Source: CAD feature listing. Evaluate the final solid. Frame: model axes, mm. Face numbers are marked on the shaded views. Round coordinates to 2 decimals unless told otherwise and drop trailing zeros. Loops run counter-clockwise (first coordinate to the right, second up) from the corner with the lowest first, then second, coordinate; pieces in that order, holes last.
(1) Section A-A, the plane y = 0. Return the cut outline in (x, z), plus the area to 4 significant figures.
(2) Mould query, pull axis X, two halves, no side actions, for the marked faces 1, 2, 3 and 4. Classes: pulls with the +X half, pulls with the -X half, needs draft (parallel to the pull), parting line crosses it, or undercut.
(3) Material intervals for probe 1 along Y at (x, z) = (0, -3); probe 2 along Z at (x, y) = (-27, -42); probe 3 along X at (y, z) = (25, -0.5), sorted ascending.
```python
from build123d import *

# Parameters (mm, degrees)
F1_DEPTH = 30
F2_R     = 75
F2_R_2   = 65
F3_DEPTH = 5


with BuildPart() as f1:
    # F0 (on Top) → F1 (new body)
    with BuildSketch(Plane.XY):
        with BuildLine():
            ThreePointArc((98.5, 75.5), (91.763456, 91.763456), (75.5, 98.5))
            Line((75.5, 98.5), (-75.5, 98.5))
            ThreePointArc((-75.5, 98.5), (-91.763456, 91.763456), (-98.5, 75.5))
            Line((-98.5, 75.5), (-98.5, -75.5))
            ThreePointArc((-98.5, -75.5), (-91.763456, -91.763456), (-75.5, -98.5))
            Line((-75.5, -98.5), (75.5, -98.5))
            ThreePointArc((75.5, -98.5), (91.763456, -91.763456), (98.5, -75.5))
            Line((98.5, -75.5), (98.5, 75.5))
        make_face()
    extrude(amount=F1_DEPTH)

    # F2 (on face) → F3 (join)
    with BuildSketch(Plane.XY):
        with BuildLine():
            Line((98.5, -75.5), (98.5, 75.5))
            ThreePointArc((98.5, 75.5), (91.763456, 91.763456), (75.5, 98.5))
            Line((75.5, 98.5), (-75.5, 98.5))
            ThreePointArc((-75.5, 98.5), (-91.763456, 91.763456), (-98.5, 75.5))
            Line((-98.5, 75.5), (-98.5, -75.5))
            ThreePointArc((-98.5, -75.5), (-91.763456, -91.763456), (-75.5, -98.5))
            Line((-75.5, -98.5), (75.5, -98.5))
            ThreePointArc((75.5, -98.5), (91.763456, -91.763456), (98.5, -75.5))
        make_face()
        Circle(F2_R, mode=Mode.SUBTRACT)
        Circle(F2_R)
        Circle(F2_R_2, mode=Mode.SUBTRACT)
    extrude(amount=-F3_DEPTH)


solid = f1.part
```
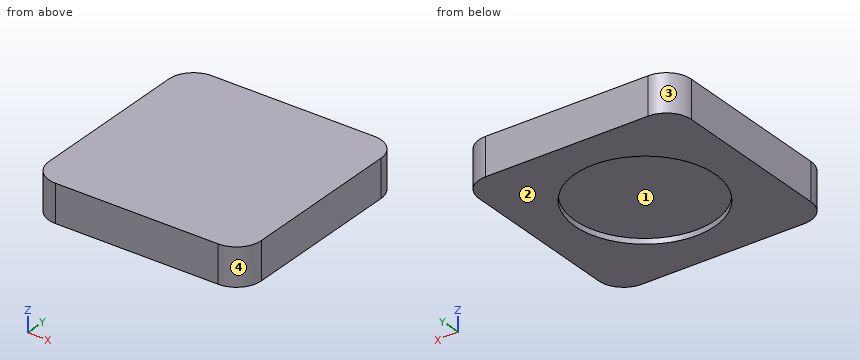
Output values:
1. outline: (-98.5, -5) - (-65, -5) - (-65, 0) - (65, 0) - (65, -5) - (98.5, -5) - (98.5, 30) - (-98.5, 30) - close
1. area: 6,245 mm2
2. face 1: undercut
2. face 2: needs draft
2. face 3: pulls with the -X half
2. face 4: pulls with the +X half
3. probe 1: y = -98.5 to -65, 65 to 98.5
3. probe 2: z = 0 to 30
3. probe 3: x = -98.5 to -60, 60 to 98.5
